Build history of the part. All positions in model axes, mm. A direction names the side the tool comes from. Give positions to 0.01 mm unless a question says otherwise; leave off trailing zeros. Loops run counter-clockwise (first coordinate to the right, second up) from the corner with the lowest first, then second, coordinate; pieces in that order, holes last. Notation, with made-up numbers: (16.25, 7.5) -> (75.25, 7.5) arc R23 ccw to (75.25, 40.5) -> close; hole circle Ø2 at (60, 7). An arc over 180 degrees is marked (long way). Answer as a JSON object with one key per item and string values. Group by question number.
Q1. Band-saw the part on A-A, the plane y = 4.5. Count the separate pieces of the cut face and the enclosed holes in it, plus the area to 3 significant figures.
Q2. Band-saw the part on C-C, the plane x = 18. Write the cut outline in (y, z).
Q3. Two-plate mould, pull along X, no slides. Class faces 1 (the cylindrical face through (-30.235, 3.131, 23.183)), 2 (the cylindrical face through (-31.303, 1.565, -1.297)), 3 (the flat face through (-1, 6.35, -1)): pulls with the +X half, pulls with the -X half, needs draft (parallel to the pull), parting line crosses it, or undercut.
Q4. Drop flat-ended pins along their axis: pin 1 (3 mm diameter, centred on y = 3.5, z = 10.5, fed in from +X); pin 2 (1 mm diameter, centred on y = 3, z = -8.5, fed in from +X); pin 3 (2 mm diameter, centred on x = -21, y = 2, fed in from -Z). Give the stop position or say it passes through.
Q5. Band-saw the part on B-B, the plane z = 17.5. Write the cut outline in (x, y), plus the area to 3 significant figures.
Q6. Wall check: probe 1 along X at (y, z) = (4, -23); probe 2 along X at (y, z) = (2.75, -24). Give the ranges that are in metal, low to high. Write a range as from..to.
Q7. Tool access for faces 4 (the cylindrical face through (24.784, 4.785, -24.344)), 5 (the cylindrical face through (31.303, 1.565, 1.297)): list every direction of +Z, -Z, +X, -X, +Y, -Y with a clear straight run to the whole face (end or side of a thin tool).
from build123d import *

# Parameters (mm, degrees)
SKETCH1_R                                      = 38.1
BOSS_EXTRUDE1_DEPTH                            = 6.35
CBORE_FOR_4_BUTTON_HEAD_CAP_SCREW1_D           = 2.8702
CBORE_FOR_4_BUTTON_HEAD_CAP_SCREW1_CBORE_D     = 4.826
CBORE_FOR_4_BUTTON_HEAD_CAP_SCREW1_CBORE_DEPTH = 3.175
CIRPATTERN1_COUNT                              = 8
SKETCH6_R                                      = 0.396875
CUT_EXTRUDE1_DEPTH                             = 7.35
CIRPATTERN2_COUNT                              = 4
SKETCH6_3_R                                    = 0.396875
CUT_EXTRUDE2_DEPTH                             = 7.35
SKETCH8_R                                      = 0.79375
CIRPATTERN4_COUNT                              = 3


with BuildPart() as part:
    # Sketch1 → Boss-Extrude1 (new body)
    with BuildSketch(Plane(origin=(0, 0, 0), x_dir=(1, 0, 0), z_dir=(0, 1, 0))):
        Circle(SKETCH1_R)
    extrude(amount=BOSS_EXTRUDE1_DEPTH)

    # CBORE for _4 Button Head Cap Screw1 (through all)
    with Locations(Plane(origin=(0, 0, 0), x_dir=(-1, 0, 0), z_dir=(0, -1, 0))):
        with Locations((0, -33.3375)):
            cbore_for_4_button_head_cap_screw1 = CounterBoreHole(CBORE_FOR_4_BUTTON_HEAD_CAP_SCREW1_D / 2, CBORE_FOR_4_BUTTON_HEAD_CAP_SCREW1_CBORE_D / 2, CBORE_FOR_4_BUTTON_HEAD_CAP_SCREW1_CBORE_DEPTH)

    # CirPattern1: CBORE for _4 Button Head Cap Screw1 ×8 about axis
    cirpattern1_axis = Axis((0, 0, 0), (0, 1, 0))
    for i in range(1, CIRPATTERN1_COUNT):
        add(cbore_for_4_button_head_cap_screw1.rotate(cirpattern1_axis, i * 360 / CIRPATTERN1_COUNT), mode=Mode.SUBTRACT)

    # Sketch6 → Cut-Extrude1 (cut, through all)
    with BuildSketch(Plane.XZ):
        with Locations((0.805087789, -1.726516334)):
            Circle(SKETCH6_R)
        with Locations((1.726516334, -0.805087789)):
            Circle(SKETCH6_R)
    cut_extrude1 = extrude(amount=-CUT_EXTRUDE1_DEPTH, mode=Mode.SUBTRACT)

    # CirPattern2: Cut-Extrude1 ×4 about axis
    cirpattern2_axis = Axis((-0.000283867, 0, 0.000283867), (0, 1, 0))
    for i in range(1, CIRPATTERN2_COUNT):
        add(cut_extrude1.rotate(cirpattern2_axis, i * 360 / CIRPATTERN2_COUNT), mode=Mode.SUBTRACT)

    # Sketch6_3 → Cut-Extrude2 (cut, through all)
    with BuildSketch(Plane.XZ):
        Circle(SKETCH6_3_R)
    extrude(amount=-CUT_EXTRUDE2_DEPTH, mode=Mode.SUBTRACT)

    # Cut-Sweep2: sweep along a curve in space
    with BuildLine() as cut_sweep2_path:
        Line((0, 6.35, -8.509), (0, 0, -6.35))
    # Sketch8 → Cut-Sweep2 (sweep, cut)
    with BuildSketch(Plane(origin=(0, 6.35, 0), x_dir=(1, 0, 0), z_dir=(0, 1, 0))):
        with Locations((0, 8.509)):
            Circle(SKETCH8_R)
    cut_sweep2 = sweep(path=cut_sweep2_path.line, mode=Mode.SUBTRACT)

    # CirPattern4: Cut-Sweep2 ×3 about axis
    cirpattern4_axis = Axis((0, 6.35, 0), (0, -1, 0))
    for i in range(1, CIRPATTERN4_COUNT):
        add(cut_sweep2.rotate(cirpattern4_axis, i * 360 / CIRPATTERN4_COUNT), mode=Mode.SUBTRACT)


solid = part.part
Worked answers:
{
 "1": {"separate pieces": "1", "enclosed holes": "20", "area": "4,500 mm2"},
 "2": {"outline": "(0, -33.58) -> (6.35, -33.58) -> (6.35, 33.58) -> (0, 33.58) -> close"},
 "3": {"face 1": "parting line crosses it", "face 2": "undercut", "face 3": "needs draft"},
 "4": {"pin 1": "x = 37.02", "pin 2": "x = 37.25", "pin 3": "z = -32.43"},
 "5": {"outline": "(-33.84, 0) -> (33.84, 0) -> (33.84, 6.35) -> (-33.84, 6.35) -> close", "area": "430 mm2"},
 "6": {"probe 1": "-30.37..-24.89, -22.26..22.26, 24.89..30.37", "probe 2": "-29.59..-25.95, -21.2..21.2, 25.95..29.59"},
 "7": {"face 4": "+Y, -Y", "face 5": "-Y"}
}
